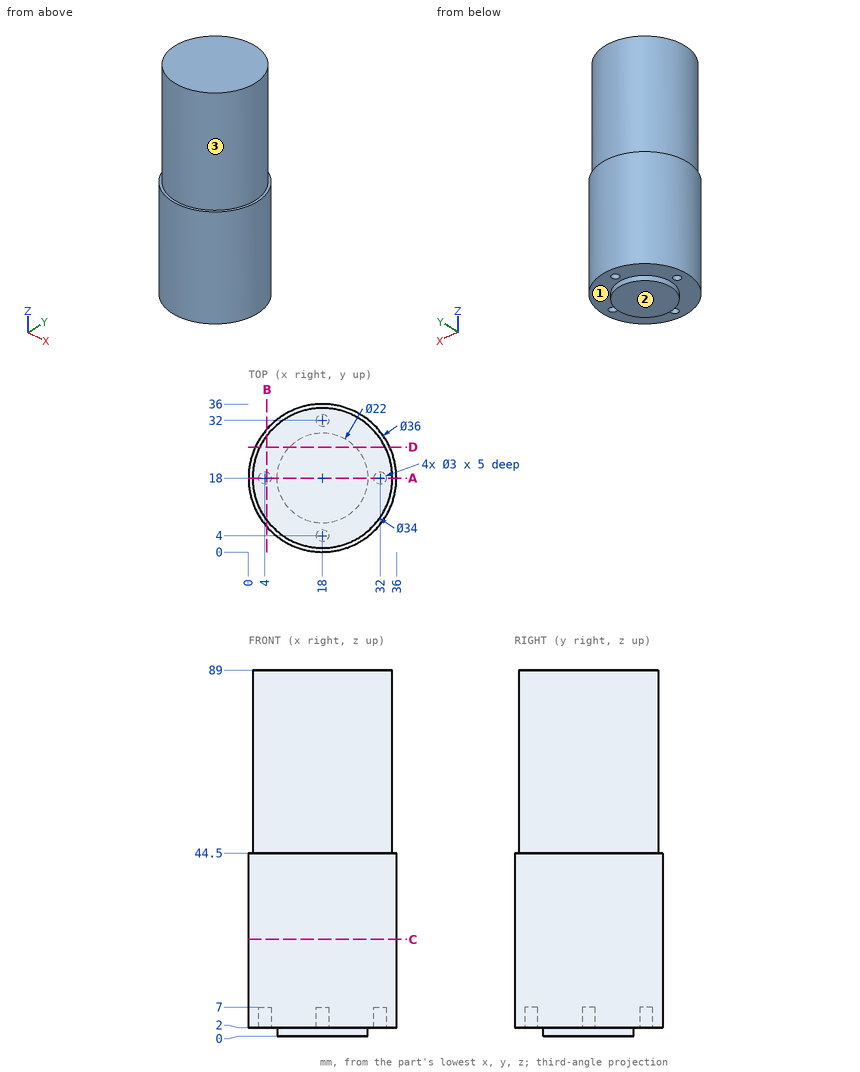
Geometry check sheet. Reference: drawing and pictorial views, mm from the part's lowest x, y, z. A direction names the side the tool comes from. Round coordinates to 2 decimals unless told otherwise and drop trailing zeros. Loops run counter-clockwise (first coordinate to the right, second up) from the corner with the lowest first, then second, coordinate; pieces in that order, holes last. Notation, with made-up numbers: (89.25, -1) - (130.25, -1) arc R6 cw to (130.25, 10) - close; hole circle Ø5 at (-23.5, 76). An arc over 180 degrees is marked (long way). Answer as CSV lines item,"result".
(1) Cross-section at A-A, the plane y = 18. Enter the section's corners in (x, z), and give its area (3 significant figures).
Output values:
outline,"(0, 2) - (2.5, 2) - (2.5, 7) - (5.5, 7) - (5.5, 2) - (7, 2) - (7, 0) - (29, 0) - (29, 2) - (30.5, 2) - (30.5, 7) - (33.5, 7) - (33.5, 2) - (36, 2) - (36, 44.5) - (35, 44.5) - (35, 89) - (1, 89) - (1, 44.5) - (0, 44.5) - close"
area,"3,060 mm²"
(2) Material ranges on line 1 along Z through (x, y) = (27, 10); line 2 along Y through (x, z) = (25, 75); line 3 along Y through (x, z) = (4, 4.4), recorded low to high.
Output values:
line 1,"z = 2 to 89"
line 2,"y = 2.51 to 33.49"
line 3,"y = 6.69 to 16.5, 19.5 to 29.31"
(3) Set-up check for the marked faces 1, 2 and 3: record each of +Z, -Z, +X, -X, +Y, -Y from which the full face is reachable in a straight line by a thin tool's end or side.
Output values:
face 1,"-Z"
face 2,"-Z, +X, -X, +Y, -Y"
face 3,"+Z"
(4) Cross-section at D-D, the plane y = 25.5. Enter the section's corners in (x, z).
Output values:
outline,"(1.64, 2) - (9.95, 2) - (9.95, 0) - (26.05, 0) - (26.05, 2) - (34.36, 2) - (34.36, 44.5) - (33.26, 44.5) - (33.26, 89) - (2.74, 89) - (2.74, 44.5) - (1.64, 44.5) - close"
(5) Cross-section at C-C, the plane z = 23.5. Enter the section's corners in (x, y).
Output values:
outline,"circle Ø36 at (18, 18)"
(6) Cross-section at B-B, the plane x = 4.5. Enter the section's corners in (y, z), and give its area (3 significant figures).
Output values:
outline,"(6.09, 2) - (16.59, 2) - (16.59, 7) - (19.41, 7) - (19.41, 2) - (29.91, 2) - (29.91, 44.5) - (28.33, 44.5) - (28.33, 89) - (7.67, 89) - (7.67, 44.5) - (6.09, 44.5) - close"
area,"1,920 mm²"
(7) Depth check by flat-ended pin: pin 1 Ø4 at (y, z) = (12.5, 30.5) entering from +X; pin 2 Ø3.5 at (x, y) = (18.5, 32.5) entering from -Z; pin 3 Ø5 at (y, z) = (28, 37) entering from +X. Enter the tip coordinate at first touch or a pass-through.
Output values:
pin 1,"stops at x = 35.66"
pin 2,"stops at z = 2"
pin 3,"stops at x = 34.36"
